Autodesk Inventor part; units mm, degrees
ref_plane "YZ Plane" through (0, 0, 0) normal (1, 0, 0) x (0, 1, 0)
ref_plane "XZ Plane" through (0, 0, 0) normal (0, 1, 0) x (-1, 0, 0)
ref_plane "XY Plane" through (0, 0, 0) normal (0, 0, 1) x (1, 0, 0)
sketch "Sketch1" plane through (0, 0, 0) normal (0, 1, 0) x (-1, 0, 0)
  line L0 (8.5074, -53.6851) -> (-102.7512, -53.6851) construction
  line L1 (-102.7512, -53.6851) -> (-102.7512, 0.3149) construction
  line L2 (-102.7512, 0.3149) -> (8.5074, 0.3149) construction
  line L3 (8.5074, 0.3149) -> (8.5074, -53.6851) construction
  line L4 (0, 0) -> (-101.6, 0)
  line L5 (-101.6, 0) -> (-101.6, -53.34)
  line L6 (-101.6, -53.34) -> (0, -53.34)
  line L7 (0, -53.34) -> (0, 0)
  circle A0 centre (-15.24, -50.8) radius 1.75
  circle A1 centre (-13.97, -2.54) radius 1.75
  circle A2 centre (-90.17, -50.8) radius 1.75
  circle A3 centre (-96.52, -2.54) radius 1.75
  line L8 (8.5074, -43.64) -> (-9, -43.64)
  line L9 (-9, -43.64) -> (-9, -31.74)
  line L10 (-9, -31.74) -> (8.5074, -31.74)
  line L11 (8.5074, -31.74) -> (8.5074, -43.64)
  line L12 (4.072, -12) -> (-12.22, -12)
  line L13 (-12.22, -12) -> (-12.22, -2.54)
  line L14 (-12.22, -2.54) -> (4.072, -2.54)
  line L15 (4.072, -2.54) -> (4.072, -12)
  line L16 (-26, -3) -> (-93, -3)
  line L17 (-93, -3) -> (-93, 0)
  line L18 (-93, 0) -> (-26, 0)
  line L19 (-26, 0) -> (-26, -3)
  line L20 (-93, -53.34) -> (-99, -53.34)
  line L21 (-99, -53.34) -> (-99, -5)
  line L22 (-99, -5) -> (-93, -5)
  line L23 (-93, -5) -> (-93, -53.34)
  line L24 (-18, -52) -> (-88, -52)
  line L25 (-88, -52) -> (-88, -49.3951)
  line L26 (-88, -49.3951) -> (-18, -49.3951)
  line L27 (-18, -49.3951) -> (-18, -52)
  line L28 (-97.4785, -53.34) -> (-100, -51.1451)
  line L29 (-100, -51.1451) -> (-100, -41)
  line L30 (-100, -41) -> (-101.6, -39)
  line L31 (-99.1411, 0) -> (-101.6, -2.8248)
  point P0 (-99, -52.0156)
  point P1 (-26, 0)
  dimension "d37" = 3.5
  dimension "d3" = 101.6
  dimension "d6" = 53.34
  dimension "d27" = 54
  dimension "d32" = 3.5
  dimension "d35" = 15.24
  dimension "d38" = 2.54
  dimension "d40" = 13.97
  dimension "d41" = 3.5
  dimension "d42" = 3.5
  dimension "d43" = 90.17
  dimension "d45" = 2.54
  dimension "d46" = 2.54
  dimension "d48" = 96.52
  dimension "d69" = 8.5074
  dimension "d70" = 9.7
  dimension "d71" = 11.9
  dimension "d73" = 2.54
extrude "Extrusion1" add sketch "Sketch1" along normal blind 2 contours L7 L14 L13 L12 L10 L9 L8 L6 L23 L22 L21 L28 L29 L30 L5 L31 L4 L17 L16 L19 | L19 L16 L17 L4 | L7 L12 L13 L14 | L7 L8 L9 L10 | L6 L28 L21 L22 L23 | L24 L25 L26 L27
sketch "Sketch2" plane through (0, 2, 0) normal (0, 1, 0) x (1, 0, 0)
  line L0 (-8.4913, 53.8189) -> (102.7673, 53.8189) construction
  line L1 (102.7673, 53.8189) -> (102.7673, -0.1811) construction
  line L2 (102.7673, -0.1811) -> (-8.4913, -0.1811) construction
  line L3 (-8.4913, -0.1811) -> (-8.4913, 53.8189) construction
  point P0 (0, 0)
  dimension "d60" = 54
extrude "Extrusion2" add sketch "Sketch1" along normal blind 15 contours L19 L16 L17 L4 | L14 L15 L12 L7 | L7 L12 L13 L14 | L10 L11 L8 L7 | L7 L8 L9 L10 | L6 L28 L21 L22 L23 | L24 L25 L26 L27
fillet "Fillet1" radius 4 2 edges at (4.074, 15, -2.54) (4.074, 15, -12)
properties part number "arduinomega"
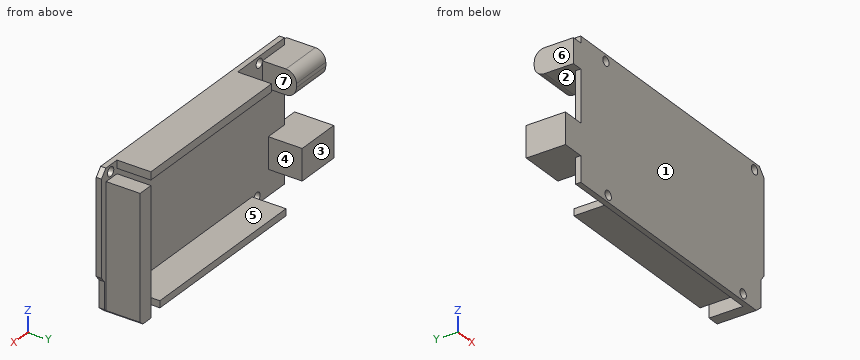
Verification items for the finished model (mm, model axes). Face numbers are marked on the shaded views. A direction names the side the tool comes from. Round coordinates to 2 decimals unless told otherwise and drop trailing zeros. Write each loop counter-clockwise with the first axis right and the second up, starting at its lowest first coordinate (ties: lowest second). Pieces come first, ordered by that corner, then holes. Notation, with made-up numbers: (58, -10) -> (110, -10) arc R27 ccw to (110, 13) -> close; hole circle Ø4 at (74.5, 39). An arc over 180 degrees is marked (long way). Write each question's results on one line, items separated by ' | '. Start each with the question number.
1. Cross-section at D-D (z = -47.5). Enter the section's corners in (x, y), then the cut area to 3 significant figures.
2. Depth check by flat-ended pin: P1, Ø1.5, axis at x = 28.5, y = 7, coming from the -Z side; P2, Ø5.5, axis at x = 4.5, y = 7, coming from the +Z side; P3, Ø8, axis at x = 89.5, z = -34.5, coming from the -Y side; P4, Ø2.5, axis at y = 9, z = -2, coming from the -X side. Enter the tip coordinate at first touch or a pass-through.
3. Cross-section at C-C (x = 46.5). Enter the section's corners in (y, z), then the cut area to 3 significant figures.
4. Cross-section at A-A (y = 3). Enter the section's corners in (x, z), then the cut area to 3 significant figures.
5. Material ranges on probe 1 along Z at (x, y) = (7, 10); probe 2 along Z at (x, y) = (13.97, 1.55); probe 3 along Z at (x, y) = (96.52, 1.4), recorded low to high. Write a range as from..to.
6. Cross-section at B-B (x = 90.17). Enter the section's corners in (y, z).
7. Draft check along Y on the marked faces 1, 2 and 3. Enter one of: +Y half, -Y half, draft (parallel to the pull), parting line (faces both ways), or undercut.
8. Set-up check for the marked faces 4, 5, 6 and 7: record each of +Z, -Z, +X, -X, +Y, -Y from which the full face is reachable in a straight line by a thin tool's end or side.
Solutions:
1) outline: (0, 0) -> (100, 0) -> (100, 2) -> (99, 2) -> (99, 15) -> (93, 15) -> (93, 2) -> (0, 2) -> close | area: 278 mm2
2) P1: stops at z = -52 | P2: stops at z = -2.54 | P3: stops at y = 0 | P4: stops at x = -4.07
3) outline: (0, -53.34) -> (2, -53.34) -> (2, -52) -> (15, -52) -> (15, -49.4) -> (2, -49.4) -> (2, -3) -> (15, -3) -> (15, 0) -> (0, 0) -> close | area: 180 mm2
4) outline: (-8.51, -43.64) -> (9, -43.64) -> (9, -31.74) -> (-8.51, -31.74) -> close; (-4.07, -12) -> (12.22, -12) -> (12.22, -2.54) -> (-4.07, -2.54) -> close; (18, -52) -> (88, -52) -> (88, -49.4) -> (18, -49.4) -> close; (26, -3) -> (93, -3) -> (93, 0) -> (26, 0) -> close; (93, -53.34) -> (97.48, -53.34) -> (99, -52.02) -> (99, -5) -> (93, -5) -> close | area: 1,030 mm2
5) probe 1: z = -43.64..-31.74, -12..-2.54 | probe 2: z = -53.34..-52, -49.6..-4.29, -0.79..0 | probe 3: z = -53.34..-4.29, -0.79..0
6) outline: (0, -53.34) -> (2, -53.34) -> (2, -52.55) -> (0, -52.55) -> close; (0, -49.05) -> (2, -49.05) -> (2, -3) -> (15, -3) -> (15, 0) -> (0, 0) -> close
7) face 1: -Y half | face 2: draft | face 3: +Y half
8) face 4: -Z, +Y | face 5: -X, +Y | face 6: +Z, -X, +Y, -Y | face 7: +Z, -Z, +Y
